Autodesk Inventor part; units mm, degrees
ref_plane "YZ Plane" through (0, 0, 0) normal (1, 0, 0) x (0, 1, 0)
ref_plane "XZ Plane" through (0, 0, 0) normal (0, 1, 0) x (-1, 0, 0)
ref_plane "XY Plane" through (0, 0, 0) normal (0, 0, 1) x (1, 0, 0)
sketch "Sketch1" plane through (0, 0, 0) normal (0, 0, 1) x (1, 0, 0)
  line L0 (-60.8901, 2.539) -> (2.3555, 66.2618)
  line L1 (2.3555, 66.2618) -> (65.601, 2.539)
  line L2 (65.601, 2.539) -> (2.3555, -61.1838)
  line L3 (2.3555, -61.1838) -> (-60.8901, 2.539)
  circle A0 centre (2.3555, 66.2618) radius 3
  circle A1 centre (-60.8901, 2.539) radius 3
  circle A2 centre (2.3555, -61.1838) radius 3
  circle A3 centre (65.601, 2.539) radius 3
  line L4 (-2.6445, 61.2618) -> (7.3555, 71.2618) construction
  line L5 (7.3555, 61.2618) -> (-2.6445, 71.2618) construction
  line L6 (-65.8901, -2.461) -> (-55.8901, 7.539) construction
  line L7 (-55.8901, -2.461) -> (-65.8901, 7.539) construction
  circle A4 centre (2.3555, 2.539) radius 100
  circle A5 centre (2.3555, 2.539) radius 70
  line L8 (65.601, 2.539) -> (-60.889, 2.539)
  line L9 (-70.889, -7.461) -> (-70.889, 12.539)
  line L10 (-70.889, 12.539) -> (-50.889, 12.539)
  line L11 (-50.889, 12.539) -> (-50.889, -7.461)
  line L12 (-50.889, -7.461) -> (-70.889, -7.461)
  line L13 (-70.889, -7.461) -> (-50.889, 12.539) construction
  line L14 (-70.889, 12.539) -> (-50.889, -7.461) construction
  line L15 (55.601, -7.461) -> (55.601, 12.539)
  line L16 (55.601, 12.539) -> (75.601, 12.539)
  line L17 (75.601, 12.539) -> (75.601, -7.461)
  line L18 (75.601, -7.461) -> (55.601, -7.461)
  line L19 (55.601, -7.461) -> (75.601, 12.539) construction
  line L20 (55.601, 12.539) -> (75.601, -7.461) construction
  line L21 (2.3555, 66.2618) -> (2.3555, 56.2618)
  line L22 (2.3555, 56.2618) -> (-7.5696, 56.2618)
  line L23 (-7.5696, 56.2618) -> (-7.5696, 71.8318)
  line L24 (2.3555, 56.2618) -> (12.2806, 56.2618)
  line L25 (12.2806, 56.2618) -> (12.2806, 71.8318)
  line L26 (2.3555, -61.1838) -> (2.3555, -51.1838)
  line L27 (2.3555, -51.1838) -> (-7.5696, -51.1838)
  line L28 (-7.5696, -66.7538) -> (-7.5696, -51.1838)
  line L29 (2.3555, -51.1838) -> (12.2806, -51.1838)
  line L30 (12.2806, -51.1838) -> (12.2806, -66.7538)
  line L31 (-50.965, 12.539) -> (55.601, 12.539)
  line L32 (55.601, 12.539) -> (55.601, -7.461)
  line L33 (55.601, -7.461) -> (-50.965, -7.461)
  line L34 (-50.965, -7.461) -> (-50.965, 12.539)
  line L35 (12.2806, -51.1838) -> (-7.5696, -51.1838)
  line L36 (-7.5696, -51.1838) -> (-7.5696, 56.2618)
  line L37 (-7.5696, 56.2618) -> (12.2806, 56.2618)
  line L38 (12.2806, 56.2618) -> (12.2806, -51.1838)
  circle A6 centre (2.3555, 2.539) radius 69.5
  circle A7 centre (2.3555, 2.539) radius 7
  line L39 (2.3555, 2.539) -> (24.5805, 2.539)
  circle A8 centre (24.5805, 2.539) radius 2
  line L40 (2.3555, 2.539) -> (21.6029, -8.5735)
  circle A9 centre (2.3555, 2.539) radius 29.21
  circle A10 centre (21.6029, -8.5735) radius 3.175
  circle A11 centre (2.3555, 24.764) radius 3.175
  circle A12 centre (-16.892, -8.5735) radius 3.175
  point P0 (0, 0)
  point P1 (-60.8901, 2.539)
  point P2 (-66.9266, 12.539)
  point P3 (-66.9266, -7.461)
  point P4 (-50.965, -7.461)
  point P5 (12.2806, 12.539)
  point P6 (-7.5696, 12.539)
  point P7 (-50.889, -7.461)
  point P8 (-7.5696, -7.461)
  point P9 (12.2806, -7.461)
  point P10 (71.6375, -7.461)
  point P11 (71.6375, 12.539)
  point P12 (12.2806, 71.3266)
  point P13 (-7.5696, 71.3266)
  point P14 (-7.5696, -66.2487)
  point P15 (12.2806, -66.2487)
  point P16 (71.1323, -7.461)
  point P17 (71.1323, 12.539)
  point P18 (-66.4214, 12.539)
  point P19 (-66.4214, -7.461)
  point P20 (-7.5696, 30.0111)
  point P21 (-25.0895, 12.539)
  point P22 (-25.0895, -7.461)
  point P23 (-7.5696, -24.9331)
  point P24 (12.2806, -24.9331)
  point P25 (29.8004, -7.461)
  point P26 (29.8004, 12.539)
  point P27 (12.2806, 30.0111)
  dimension "d0" = 6
  dimension "d1" = 6
  dimension "d2" = 6
  dimension "d3" = 6
  dimension "d8" = 200
  dimension "d9" = 140
  dimension "d10" = 126.49
  dimension "d11" = 20
  dimension "d12" = 20
  dimension "d13" = 20
  dimension "d14" = 20
  dimension "d18" = 10
  dimension "d19" = 10
  dimension "d22" = 139
  dimension "d24" = 14
  dimension "d25" = 22.225
  dimension "d26" = 4
  dimension "d31" = 22.225
  dimension "d32" = 30
  dimension "d33" = 58.42
  dimension "d34" = 6.35
  dimension "d37" = 360
extrude "Extrusion1" add sketch "Sketch1" along normal blind 2 contours L34 L8 A1 L0 | L0 A1 L3 L12 A6 L10 | L10 L11 L8 L34 | L23 A6 L25 L1 A0 L0 | L0 A0 L21 L22 | L22 L24 L38 A9 L36 | L31 A9 L8 L11 | L34 L3 A1 L8 | L8 L11 L12 L34 | L21 A0 L1 L24 | A9 L38 L31 L36 | L36 L31 A9 | L8 A9 L33 L11 | L31 L36 L8 A9 | L31 L38 L8 A7 L36 | A9 L31 L38 | L8 L36 L33 A12 A9 | L28 L3 A2 L2 L30 A6 | L27 L26 A2 L3 | L36 A9 L38 L29 L27 | L16 A6 L18 L2 A3 L1 | L1 A3 L8 L15 L16 | L31 A9 L8 A8 L38 | L8 A7 L40 L38 L33 L36 | L31 L15 L8 A9 | L33 A12 L36 A9 | L29 L2 A2 L26 | L36 L33 L38 A9 | L38 L40 A7 L8 | L8 A8 A9 L33 A10 L40 L38 | A7 L8 | L8 L40 A7 | L8 L15 L33 A9 | L38 L33 A10 A9 | A3 L2 L18 L15 L8 | A8 L8 | L8 A8 | A7 L40 L8 | L40 A10 L33 L38
fillet "Fillet2" radius 6.35 8 edges at (29.8004, 12.539, 1) (12.2806, 30.0111, 1) (-25.0895, 12.539, 1) (-7.5696, 30.0111, 1) (-7.5696, -24.9331, 1) (-25.0895, -7.461, 1) (12.2806, -24.9331, 1) (29.8004, -7.461, 1)
properties part number "steering sheet"
Geometry check sheet. Reference: the model listing, model coordinates, mm. Round coordinates to 2 decimals unless told otherwise and drop trailing zeros. Loops run counter-clockwise (first coordinate to the right, second up) from the corner with the lowest first, then second, coordinate; pieces in that order, holes last. Notation, with made-up numbers: (-22, -24.75) -> (18, -24.75) arc R19 ccw to (18, -19.75) -> close; hole circle Ø5 at (2, -1.5). An arc over 180 degrees is marked (long way). Use a Markdown table: item, result.
(1) Sectioned sample at B-B (y = -56). Enter the section's corners in (x, z).
Calculated:
| item | result |
|---|---|
| outline | (-7.57, 0) -> (12.28, 0) -> (12.28, 2) -> (-7.57, 2) -> close |
(2) Mould release check, pull along Y, two halves, no side actions. Record for faces 1 (the cylindrical face through (62.604, 2.407, 0.986)), 2 (the flat face through (2, -2, 2)), 3 (the cylindrical face through (-25.96, 13.44, 1.01)): released by +Y, released by -Y, zero draft, split by the parting line, or undercut.
Calculated:
| item | result |
|---|---|
| face 1 | undercut |
| face 2 | zero draft |
| face 3 | released by +Y |
(3) Go/stop test with flat-tipped pins: P1, Ø5, axis at x = 2.36, y = 66.26, coming from the +Z side; P2, Ø0.6, axis at x = 44.5, z = 1, coming from the -Y side; P3, Ø1, axis at y = 31, z = 1.5, coming from the -X side; P4, Ø0.6, axis at y = 55, z = 0.5, coming from the +X side. Record where each tip stops, or that it passes through.
Calculated:
| item | result |
|---|---|
| P1 | through |
| P2 | y = -7.46 |
| P3 | x = -8.73 |
| P4 | x = 12.28 |
(4) Sectioned sample at A-A (z = 0.5). Give the number of separate pieces and of enclosed holes in the cut face, then the cut area to 3 significant figures.
Calculated:
| item | result |
|---|---|
| separate pieces | 1 |
| enclosed holes | 7 |
| area | 5,730 mm² |
(5) Sectioned sample at C-C (x = -36). Enter the section's corners in (y, z).
Calculated:
| item | result |
|---|---|
| outline | (-7.46, 0) -> (12.54, 0) -> (12.54, 2) -> (-7.46, 2) -> close |
(6) Scan lines: probe 1 along Y at (x, z) = (2.5, 0.9); probe 2 along X at (y, z) = (-10, 1.4); probe 3 along X at (y, z) = (-47.5, 1.05). Record each from-to range of solid material in increasing order.
Calculated:
| item | result |
|---|---|
| probe 1 | -66.96 to -64.18, -58.19 to 21.59, 27.94 to 63.27, 69.26 to 72.04 |
| probe 2 | -24.14 to -19.73, -14.06 to 18.77, 24.44 to 28.85 |
| probe 3 | -7.57 to 12.28 |
